Design review of the part built by this model. Coordinates are the model's own, in mm. A direction names the side the tool comes from. Round coordinates to 2 decimals unless told otherwise and drop trailing zeros. Order: outer loops, then holes, each group sorted by start corner. A loop starts at its lowest first (then second) coordinate and runs counter-clockwise, first axis right, second up. Notation, with made-up numbers: (17, 30) - (71, 30) arc R13 ccw to (71, 51) - close; hole circle Ø5 at (74.25, -7). An arc over 180 degrees is marked (long way). Write item = value, one per line.
from build123d import *

# Parameters (mm, degrees)
SKETCH1_R                 = 16
SKETCH1_R_2               = 3
BOSS_EXTRUDE1_DEPTH       = 4.25
CUT_EXTRUDE1_REACH        = 26.023
CUT_EXTRUDE1_START_RADIUS = 16
CUT_EXTRUDE1_END_RADIUS   = 16
SKETCH2_W                 = 1
SKETCH2_H                 = 3


with BuildPart() as part:
    # Sketch1 → Boss-Extrude1 (new body)
    with BuildSketch(Plane(origin=(0, 0, 0), x_dir=(1, 0, 0), z_dir=(0, 1, 0))):
        with Locations(Location((0, 0, 0), (0, 0, 270))):
            Circle(SKETCH1_R)
        with Locations(Location((0, 0, 0), (0, 0, 270))):
            Circle(SKETCH1_R_2, mode=Mode.SUBTRACT)
    extrude(amount=BOSS_EXTRUDE1_DEPTH)

    # Cut-Extrude1: from a cylinder face, 26.023 long prism both ways, kept between that surface and its translate by the depth
    cut_extrude1_start = Plane(origin=(0, 2.75, 0), z_dir=(0, -1, 0)) * Cylinder(CUT_EXTRUDE1_START_RADIUS, 85.046, mode=Mode.PRIVATE)
    cut_extrude1_end = Plane(origin=(0, 2.75, -1), z_dir=(0, -1, 0)) * Cylinder(CUT_EXTRUDE1_END_RADIUS, 85.046, mode=Mode.PRIVATE)
    # Sketch2 → Cut-Extrude1 (cut, from a surface)
    with BuildSketch(Plane.XY, mode=Mode.PRIVATE) as cut_extrude1_sk1:
        with Locations((0, 2.75)):
            Rectangle(SKETCH2_W, SKETCH2_H)
    cut_extrude1_tool1 = extrude(cut_extrude1_sk1.sketch, amount=CUT_EXTRUDE1_REACH, both=True, mode=Mode.PRIVATE)
    add(((cut_extrude1_tool1 & cut_extrude1_start) - cut_extrude1_end).solids().sort_by_distance((0, 2.75, 15.492186))[0], mode=Mode.SUBTRACT)


solid = part.part
Item 1: Take a section at C-C, the plane y = 1.7. State the section outline as (x, z) points, and give its area (3 significant figures).
Data:
outline = (-0.5, 14.99) - (-0.5, 15.99) arc R16 ccw (long way) to (0.5, 15.99) - (0.5, 14.99) arc R16 ccw to start; hole circle Ø6 at (0, 0)
area = 775 mm2
Item 2: Take a section at D-D, the plane z = 6. State the section outline as (x, y) points.
Data:
outline = (-14.83, 0) - (14.83, 0) - (14.83, 4.25) - (-14.83, 4.25) - close
Item 3: For faces 1 (the face through (0, 3, 15)), 2 (the face through (0.9, 2.1, 2.86)), list the 3-axis set-ups (+Z, -Z, +X, -X, +Y, -Y) from which the entire face can be reached by the end or side of a thin tool; tool diameter is ignored.
Data:
face_1 = +Z, +Y
face_2 = +Y, -Y
Item 4: Take a section at B-B, the plane x = 0. State the section outline as (y, z) points, and give its area (4 significant figures).
Data:
outline = (0, -16) - (4.25, -16) - (4.25, -3) - (0, -3) - close; (0, 3) - (4.25, 3) - (4.25, 15) - (1.25, 15) - (1.25, 16) - (0, 16) - close
area = 107.5 mm2
Item 5: Take a section at A-A, the plane z = 0. State the section outline as (x, y) points.
Data:
outline = (-16, 0) - (-3, 0) - (-3, 4.25) - (-16, 4.25) - close; (3, 0) - (16, 0) - (16, 4.25) - (3, 4.25) - close
Item 6: For line 1 along X through (y, z) = (2.75, 0); line 2 along X through (y, z) = (2.75, 1); line 3 along Z through (x, y) = (1.5, 1.4), list the stretches that pass through material, from the lowest coordinate up. Write a range as [from, to].
Data:
line_1 = [-16, -3], [3, 16]
line_2 = [-15.97, -2.83], [2.83, 15.97]
line_3 = [-15.93, -2.6], [2.6, 15.93]
Item 7: The part is to be moulded in two halves that separate along X. For faces 3 (the face through (0, 1.25, 15.5)), 4 (the face through (-15.62, 2.1, -3.47)), 5 (the face through (0.2, 4.25, 3.3)), say which applies: +X half, -X half, draft (parallel to the pull), parting line (faces both ways), or undercut.
Data:
face_3 = undercut
face_4 = parting line
face_5 = draft
Item 8: Insertion check: P1, Ø2, axis at y = 4, z = -6.5, coming from the -X side (3 decimals); P2, Ø0.8, axis at x = 0, z = 15.5, coming from the +Y side. Each pin has a flat end and moves straight along its axis. Give the tip position at first contact, or say it passes through.
Data:
P1 = -15.025
P2 = 1.25
